```python
from build123d import *

# Parameters (mm, degrees)
SKETCH_1_W         = 6
SKETCH_1_H         = 6
EXTRUDE_1_DEPTH    = 40
HOLE_WIZARD_M3_1_D = 2.5
HOLE_WIZARD_M3_2_D = 2.5
FILLET_1_R         = 0.5


with BuildPart() as part:
    # 草图1 → 凸台-拉伸1 (new body)
    with BuildSketch(Plane.XY):
        Rectangle(SKETCH_1_W, SKETCH_1_H)
    extrude(amount=EXTRUDE_1_DEPTH)

    # M3 螺纹孔1 (through all)
    with Locations(Plane(origin=(0, 3, 0), x_dir=(1, 0, 0), z_dir=(0, 1, 0))):
        with Locations((0, -35), (0, -15)):
            Hole(HOLE_WIZARD_M3_1_D / 2)

    # M3 螺纹孔2 (through all)
    with Locations(Plane.ZY.offset(3)):
        with Locations((5, 0), (25, 0)):
            Hole(HOLE_WIZARD_M3_2_D / 2)

    # 圆角1
    fillet_1_edges = [part.edges().sort_by_distance(p)[0] for p in [
        (-3, 0, 40),
        (0, -3, 40),
        (3, 0, 40),
        (0, -3, 0),
        (-3, 0, 0),
        (0, 3, 0),
        (3, 0, 0),
        (0, 3, 40),
        (3, -3, 20),
        (-3, -3, 20),
        (-3, 3, 20),
        (3, 3, 20),
    ]]
    fillet(fillet_1_edges, radius=FILLET_1_R)


solid = part.part
```
Input: part model. Units: mm. Frame: model coordinates. Coordinates: 2 decimals unless noted, no trailing zeros. Write each loop counter-clockwise with the first axis right and the second up, starting at its lowest first coordinate (ties: lowest second). Pieces come first, ordered by that corner, then holes. Notation, with made-up numbers: M -7,-2.5 L 29,-2.5 A31 cw 29,33.5 Z; hole C 25.5,70.25 d9. An arc over 180 degrees is marked long. Use one line per item in the form item = value.
Q1. Section C-C (z = 15). Return loops of the section in (x, y).
Answer below:
outline = M -3,-2.5 A0.5 ccw -2.5,-3 L -1.25,-3 L -1.25,3 L -2.5,3 A0.5 ccw -3,2.5 Z; M 1.25,-3 L 2.5,-3 A0.5 ccw 3,-2.5 L 3,2.5 A0.5 ccw 2.5,3 L 1.25,3 Z
Q2. Section A-A (x = 0). Return loops of the section in (y, z), plus the area to 3 significant figures.
Answer below:
outline = M -3,0.5 A0.5 ccw -2.5,0 L 2.5,0 A0.5 ccw 3,0.5 L 3,13.75 L -3,13.75 Z; M -3,16.25 L 3,16.25 L 3,33.75 L -3,33.75 Z; M -3,36.25 L 3,36.25 L 3,39.5 A0.5 ccw 2.5,40 L -2.5,40 A0.5 ccw -3,39.5 Z; hole C 0,5 d2.5; hole C 0,25 d2.5
area = 200 mm²
Q3. Material intervals for probe 1 along Z at (x, y) = (-1.85, -0.15); probe 2 along Z at (x, y) = (0, -1.4); probe 3 along Y at (x, z) = (-0.85, 25), sorted ascending. Write a range as from..to.
Answer below:
probe_1 = 0..3.76, 6.24..23.76, 26.24..40
probe_2 = 0..13.75, 16.25..33.75, 36.25..40
probe_3 = -3..-1.25, 1.25..3
Q4. Section D-D (y = 1.8). Return loops of the section in (x, z).
Answer below:
outline = M -3,0.5 A0.5 ccw -2.5,0 L 2.5,0 A0.5 ccw 3,0.5 L 3,39.5 A0.5 ccw 2.5,40 L -2.5,40 A0.5 ccw -3,39.5 Z; hole C 0,15 d2.5; hole C 0,35 d2.5
Q5. Section B-B (y = 0). Return loops of the section in (x, z).
Answer below:
outline = M -3,0.5 A0.5 ccw -2.5,0 L 2.5,0 A0.5 ccw 3,0.5 L 3,3.75 L -3,3.75 Z; M -3,6.25 L 3,6.25 L 3,23.75 L -3,23.75 Z; M -3,26.25 L 3,26.25 L 3,39.5 A0.5 ccw 2.5,40 L -2.5,40 A0.5 ccw -3,39.5 Z; hole C 0,15 d2.5; hole C 0,35 d2.5
Q6. Draft query along X for faces 1 (the face through (0, -3, 20)), 2 (the face through (3, 0, 20)), 3 (the face through (-3, 0, 20)), 4 (the face through (-0.577, -0.042, 36.109)). Return one class per face: released by +X, released by -X, zero draft, split by the parting line, or undercut.
Answer below:
face_1 = zero draft
face_2 = released by +X
face_3 = released by -X
face_4 = undercut
